from build123d import *

# Parameters (mm, degrees)
SKETCH3_W               = 4.75
SKETCH3_H               = 5.746351638
BOSS_EXTRUDE1_DEPTH     = 0.4
BOSS_EXTRUDE2_DEPTH     = 2.375
BOSS_EXTRUDE3_DEPTH     = 2.375
CUT_EXTRUDE1_DEPTH      = 12.617443781
CUT_EXTRUDE2_DEPTH      = 10.530326191
CUT_EXTRUDE2_DEPTH_BACK = 10.530326191
WRAP1_OUTLINE_R         = 0.5
WRAP1_DEPTH             = 0.08
BOSS_EXTRUDE4_DEPTH     = 11.54


# Read off the part's stored shape, not the designer's step: Wrap1
with BuildPart() as part:
    # Sketch1 → Revolve1 (revolve)
    with BuildSketch(Plane.XY, mode=Mode.PRIVATE) as revolve1_sk:
        Polygon((-3.990566038, 0), (3.759433962, 0), (3.759433962, 3.75), (2.259433962, 3.75), (2.259433962, 2.85), (-2.490566038, 2.85), (-2.490566038, 3.75), (-3.990566038, 3.75), align=None)
    revolve(revolve1_sk.sketch.rotate(Axis((-3.990566038, 0, 0), (1, 0, 0)), 180), axis=Axis((-3.990566038, 0, 0), (1, 0, 0)))

    # Sketch3 → Boss-Extrude1 (add, symmetric)
    with BuildSketch(Plane.XY):
        with Locations((-0.115566038, -3.426824181)):
            Rectangle(SKETCH3_W, SKETCH3_H)
    extrude(amount=BOSS_EXTRUDE1_DEPTH, both=True)

    # Sketch3<7> → Boss-Extrude2 (add, symmetric)
    with BuildSketch(Plane.XY):
        Polygon((2.259433962, -0.553648362), (2.259433962, -6.3), (-2.490566038, -6.3), (-2.490566038, -0.553648362), (-3.990566038, -0.553648362), (-3.990566038, -7.8), (3.759433962, -7.8), (3.759433962, -0.553648362), align=None)
    extrude(amount=BOSS_EXTRUDE2_DEPTH, both=True)

    # Sketch5 → Boss-Extrude3 (add, symmetric)
    with BuildSketch(Plane(origin=(0, 0, 0), x_dir=(-1, 0, 0), z_dir=(0, 0, -1))):
        with BuildLine():
            Line((-0.75, -6.3), (0.75, -6.3))
            Line((0.75, -6.3), (0.75, -5.497644806))
            ThreePointArc((0.75, -5.497644806), (1.2, -4.560895106), (0.75, -3.624145406))
            Line((0.75, -3.624145406), (0.75, -2.821790212))
            Line((0.75, -2.821790212), (0.75, -1.153612006))
            Line((0.75, -1.153612006), (-0.75, -1.153612006))
            Line((-0.75, -1.153612006), (-0.75, -2.821790212))
            Line((-0.75, -2.821790212), (-0.75, -3.624145406))
            ThreePointArc((-0.75, -3.624145406), (-1.2, -4.560895106), (-0.75, -5.497644806))
            Line((-0.75, -5.497644806), (-0.75, -6.3))
        make_face()
    extrude(amount=BOSS_EXTRUDE3_DEPTH, both=True)

    # Sketch2 → Cut-Extrude1 (cut, through all)
    with BuildSketch(Plane.ZY.offset(3.990566038)):
        with BuildLine():
            Line((-0.9, 2.116601049), (-0.9, 1.05))
            ThreePointArc((-0.9, 1.05), (-0.943933983, 0.943933983), (-1.05, 0.9))
            Line((-1.05, 0.9), (-2.116601049, 0.9))
            ThreePointArc((-2.116601049, 0.9), (-2.3, 0), (-2.116601049, -0.9))
            Line((-2.116601049, -0.9), (-1.05, -0.9))
            ThreePointArc((-1.05, -0.9), (-0.943933983, -0.943933983), (-0.9, -1.05))
            Line((-0.9, -1.05), (-0.9, -2.116601049))
            ThreePointArc((-0.9, -2.116601049), (0, -2.3), (0.9, -2.116601049))
            Line((0.9, -2.116601049), (0.9, -1.05))
            ThreePointArc((0.9, -1.05), (0.943933983, -0.943933983), (1.05, -0.9))
            Line((1.05, -0.9), (2.116601049, -0.9))
            ThreePointArc((2.116601049, -0.9), (2.3, 0), (2.116601049, 0.9))
            Line((2.116601049, 0.9), (1.05, 0.9))
            ThreePointArc((1.05, 0.9), (0.943933983, 0.943933983), (0.9, 1.05))
            Line((0.9, 1.05), (0.9, 2.116601049))
            ThreePointArc((0.9, 2.116601049), (0, 2.3), (-0.9, 2.116601049))
        make_face()
    extrude(amount=-CUT_EXTRUDE1_DEPTH, mode=Mode.SUBTRACT)

    # Sketch4 → Cut-Extrude2 (cut, two sides: drawn at the far end of the back side and taken through both)
    with BuildSketch(Plane.XY.offset(-CUT_EXTRUDE2_DEPTH_BACK)):
        with BuildLine():
            Line((-1.790566038, 0.575), (1.559433962, 0.575))
            ThreePointArc((1.559433962, 0.575), (2.134433962, 0), (1.559433962, -0.575))
            Line((1.559433962, -0.575), (-1.790566038, -0.575))
            ThreePointArc((-1.790566038, -0.575), (-2.365566038, 0), (-1.790566038, 0.575))
        make_face()
    extrude(amount=CUT_EXTRUDE2_DEPTH + CUT_EXTRUDE2_DEPTH_BACK, mode=Mode.SUBTRACT)

    # Wrap1 outline → Wrap1 (add)
    with BuildSketch(Plane.XY.offset(2.375)):
        with Locations((0, -4.560895106)):
            Circle(WRAP1_OUTLINE_R)
    extrude(amount=WRAP1_DEPTH)

    # Sketch7 → Boss-Extrude4 (add)
    with BuildSketch(Plane.XZ.offset(7.8)):
        with BuildLine():
            Line((-0.9, 2.116601049), (-0.9, 0.9))
            Line((-0.9, 0.9), (-2.116601049, 0.9))
            ThreePointArc((-2.116601049, 0.9), (-2.3, 0), (-2.116601049, -0.9))
            Line((-2.116601049, -0.9), (-0.9, -0.9))
            Line((-0.9, -0.9), (-0.9, -2.116601049))
            ThreePointArc((-0.9, -2.116601049), (0, -2.3), (0.9, -2.116601049))
            Line((0.9, -2.116601049), (0.9, -0.9))
            Line((0.9, -0.9), (2.116601049, -0.9))
            ThreePointArc((2.116601049, -0.9), (2.3, 0), (2.116601049, 0.9))
            Line((2.116601049, 0.9), (0.9, 0.9))
            Line((0.9, 0.9), (0.9, 2.116601049))
            ThreePointArc((0.9, 2.116601049), (0, 2.3), (-0.9, 2.116601049))
        make_face()
    extrude(amount=BOSS_EXTRUDE4_DEPTH)


solid = part.part
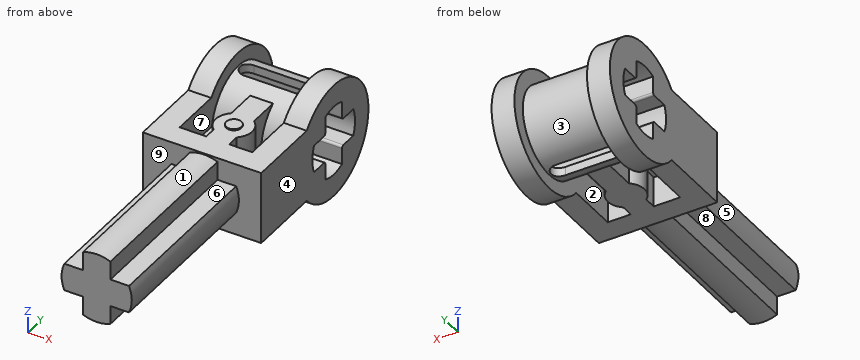
Read the model definition and answer for the solid it produces. Units are mm, in the model's axes. Face numbers are marked on the shaded views. A direction names the side the tool comes from. Round coordinates to 2 decimals unless told otherwise and drop trailing zeros. Write each loop counter-clockwise with the first axis right and the second up, starting at its lowest first coordinate (ties: lowest second). Pieces come first, ordered by that corner, then holes.
Q1. Flat-ended cylindrical pins translate along their axes: P1, Ø1, axis at x = 2.5, z = 0.5, coming from the -Y side; P2, Ø0.5, axis at x = 1, y = -5, coming from the -Z side (3 decimals); P3, Ø0.5, axis at x = -0.5, z = -2.5, coming from the +Y side; P4, Ø1.3, axis at y = -12.5, z = 1.5, coming from the -X side. Find the tip coordinate at first contact, or state that the pin passes through.
Values:
P1: stops at y = -19.34
P2: stops at z = -2.375
P3: stops at y = 1.75
P4: stops at x = -2.14
Q2. Straight lines are drawn through the part: line 1 (X direction, y = -3, z = 2.25); line 2 (Y direction, x = 3, z = 0); line 3 (Y direction, x = 1.25, z = 1). For each, find the intervals that lie inside material, in ascending order.
Values:
line 1: x = -3.99 to -2.49, -0.75 to 0.75, 2.26 to 3.76
line 2: y = -7.8 to -2.3, 2.3 to 3.75
line 3: y = -7.8 to -6.3, -2.67 to -0.91, 0.91 to 2.67
Q3. Find section C-C on y = -15. Determine the outline of the cut face in (x, z), and give its area (3 significant figures).
Values:
outline: (-2.12, -0.9) - (-0.9, -0.9) - (-0.9, -2.12) arc R2.3 ccw to (0.9, -2.12) - (0.9, -0.9) - (2.12, -0.9) arc R2.3 ccw to (2.12, 0.9) - (0.9, 0.9) - (0.9, 2.12) arc R2.3 ccw to (-0.9, 2.12) - (-0.9, 0.9) - (-2.12, 0.9) arc R2.3 ccw to start
area: 12.9 mm2
Q4. Find section D-D on z = 3.25. Determine the outline of the cut face in (x, y), and give its area (3 significant figures).
Values:
outline: (-3.99, -1.87) - (-2.49, -1.87) - (-2.49, 1.87) - (-3.99, 1.87) - close; (2.26, -1.87) - (3.76, -1.87) - (3.76, 1.87) - (2.26, 1.87) - close
area: 11.2 mm2
Q5. A tool of negligible diameter and unlimited length cuts with its end or side. For the marked faces 5, 6, 7, 8 and 9, from which of +Z, -Z, +X, -X, +Y, -Y can it reach the whole face along a straight path? Write none if from no direction.
Values:
face 5: -X, -Y
face 6: +Z, +X, -Y
face 7: none
face 8: -Z, -X, -Y
face 9: -Y
Q6. Find section B-B on x = 3. Determine the outline of the cut face in (y, z) (3 decimals).
Values:
outline: (-7.8, -2.375) - (-2.902, -2.375) arc R3.75 ccw (long way) to (-2.902, 2.375) - (-7.8, 2.375) - close; hole (-2.117, -0.9) - (-1.05, -0.9) arc R0.15 cw to (-0.9, -1.05) - (-0.9, -2.117) arc R2.3 ccw to (0.9, -2.117) - (0.9, -1.05) arc R0.15 cw to (1.05, -0.9) - (2.117, -0.9) arc R2.3 ccw to (2.117, 0.9) - (1.05, 0.9) arc R0.15 cw to (0.9, 1.05) - (0.9, 2.117) arc R2.3 ccw to (-0.9, 2.117) - (-0.9, 1.05) arc R0.15 cw to (-1.05, 0.9) - (-2.117, 0.9) arc R2.3 ccw to start
Q7. Find section A-A on z = 0. Determine the outline of the cut face in (x, y).
Values:
outline: (-3.99, -7.8) - (-2.3, -7.8) - (-2.3, -19.34) - (2.3, -19.34) - (2.3, -7.8) - (3.76, -7.8) - (3.76, -2.3) - (-3.99, -2.3) - close; (-3.99, 2.3) - (3.76, 2.3) - (3.76, 3.75) - (2.26, 3.75) - (2.26, 2.85) - (-2.49, 2.85) - (-2.49, 3.75) - (-3.99, 3.75) - close
Q8. The mould has two halves that part along X. Classify the marked faces 1, 2, 3 and 4: released by +X, released by -X, zero draft, split by the parting line, or undercut.
Values:
face 1: split by the parting line
face 2: undercut
face 3: undercut
face 4: released by +X
